```python
from build123d import *

# Parameters (mm, degrees)
F0_W          = 53.4308515489
F0_H          = 2.8585356195
F3_DEPTH      = 25
F3_DEPTH_BACK = 25


with BuildPart() as f1:
    # F0 (on Front) → F1 (revolve)
    with BuildSketch(Plane.XZ):
        with BuildLine():
            Line((-51.769964397, 0), (0, 0))
            Line((0, 0), (0, 2.8585356195))
            add(Edge.make_bspline(
                [(-51.769964397, 0), (-51.9150732548, 5.9729817036), (-48.5666547713, 9.9986232463), (-28.5664722225, 9.3824894101), (-10.8998766604, 6.9841195767), (-1.008867938, 4.4151364363), (0, 2.8585356195)],
                knots=[0, 0, 0, 0, 0.2062985932, 0.4897524386, 0.7883562467, 1, 1, 1, 1], degree=3))
        make_face()
        with Locations((26.7154257745, 1.4292678097)):
            Rectangle(F0_W, F0_H)
    revolve(axis=Axis((0.830443576, 0, 0), (-1, 0, 0)))

    # F2 (on Front) → F3 (cut, two sides)
    with BuildSketch(Plane.XZ) as f3_sk:
        with BuildLine():
            Line((55.8451525867, 3.1400402716), (45.2548848048, 3.1400402716))
            add(Edge.make_bspline(
                [(45.2548848048, 3.1400402716), (45.9080027919, 2.3053192042), (49.4573835127, 0.8682668184), (53.7558149824, 0.0506240562), (56.130883876, 0.5836136314)],
                knots=[0, 0, 0, 0, 0.4437761369, 1, 1, 1, 1], degree=3))
            Line((56.130883876, 0.5836136314), (55.8451525867, 3.1400402716))
        make_face()
        with BuildLine():
            add(Edge.make_bspline(
                [(45.2548848048, -3.1400402716), (45.9080027919, -2.3053192042), (49.4573835127, -0.8682668184), (53.7558149824, -0.0506240562), (56.130883876, -0.5836136314)],
                knots=[0, 0, 0, 0, 0.4437761369, 1, 1, 1, 1], degree=3))
            Line((45.2548848048, -3.1400402716), (55.8273755014, -3.5082600079))
            Line((55.8273755014, -3.5082600079), (56.130883876, -0.5836136314))
        make_face()
    extrude(amount=-F3_DEPTH, mode=Mode.SUBTRACT)
    extrude(f3_sk.sketch, amount=F3_DEPTH_BACK, mode=Mode.SUBTRACT)


solid = f1.part
```
Design review of the part built by this model. Coordinates are the model's own, in mm. Give positions to 0.01 mm unless a question says otherwise; leave off trailing zeros. Order: outer loops, then holes, each group sorted by start corner. A loop starts at its lowest first (then second) coordinate and runs counter-clockwise, first axis right, second up. Notation, with made-up numbers: (58.25, -29) -> (110.25, -29) arc R19 ccw to (110.25, -12) -> close; hole circle Ø11 at (43, 78.25). An arc over 180 degrees is marked (long way). Write each question's results on one line, items separated by ' | '. Start each with the question number.
Q1. Add section A-A on x = 25.5. Give the boundary of the cut face in (y, z), and give its area (3 significant figures).
Q2. For pin 1 (4 mm diameter, centred on x = 19, z = -4, fed in from -Y); pin 2 (4 mm diameter, centred on y = 4.5, z = 6.5, fed in from -X); pin 3 (1.5 mm diameter, centred on x = -29, y = 4.5, fed in from -Z), all flat-tipped, find the tip position at first contact; note any pin that passes through.
Q3. Wall thickness on L1, parallel to Y at x = -12, z = 6.25; L2, parallel to Z at x = -39.5, y = 6.75; L3, parallel to Y at x = -22.5, z = -4.5: over which ranges is each line inside the solid? List them lowest first. Write a range as from..to.
Found:
1) outline: circle Ø5.72 at (0, 0) | area: 25.7 mm2
2) pin 1: stops at y = -2.04 | pin 2: stops at x = -50.96 | pin 3: stops at z = -8.25
3) L1: y = -2.83..2.83 | L2: z = -6.69..6.69 | L3: y = -7.12..7.12
